Geometry: final body of the model. Coordinates: model frame, mm. Face numbers are marked on the shaded views. Give positions to 0.01 mm unless a question says otherwise; leave off trailing zeros. Write each loop counter-clockwise with the first axis right and the second up, starting at its lowest first coordinate (ties: lowest second). Pieces come first, ordered by that corner, then holes. Notation, with made-up numbers: M -27,76 L 30,76 A27 ccw 30,101 Z; hole C 13.25,-30 d9. An arc over 180 degrees is marked long. Use a Markdown table: item, result. Add a question column.
1) Section A-A on y = 0. Return the cut outline in (x, z).
2) Line query: line 1 (Z direction, x = 3, y = 1.2); line 2 (X direction, y = 1, z = 0.85); line 3 (X direction, y = -0.15, z = 1.1). Output: solid intervals per line, ascending.
3) Draft query along X for the marked faces 1, 2 and 3. Return one class per face: +X half, -X half, draft (parallel to the pull), parting line (faces both ways), or undercut.
4) Section C-C on z = 0.35. Return the cut outline in (x, y).
5) Pin query (flat end, axial travel): pin 1 (0.9 mm diameter, centred on x = 2.5, y = 0, fed in from +Z). Return the tip coordinate at first contact, or that it passes through.
6) Section D-D on x = 0.75. Return the cut outline in (y, z), then the cut area to 3 significant figures.
7) Section B-B on x = 8.75. Return the cut outline in (y, z).
Autodesk Inventor part; units mm, degrees
ref_plane "YZ Plane" through (0, 0, 0) normal (1, 0, 0) x (0, 1, 0)
ref_plane "XZ Plane" through (0, 0, 0) normal (0, 1, 0) x (-1, 0, 0)
ref_plane "XY Plane" through (0, 0, 0) normal (0, 0, 1) x (1, 0, 0)
sketch "草图1" plane through (0, 0, 0) normal (0, 0, 1) x (1, 0, 0)
  line L0 (-8.5, 0) -> (8.5, 0) construction
  line L1 (-8.5, -1.5) -> (8.5, -1.5)
  line L2 (8.5, 1.5) -> (-8.5, 1.5)
  arc A0 (-8.5, 1.5) -> (-8.5, -1.5) centre (-8.5, 0) ccw
  arc A1 (8.5, -1.5) -> (8.5, 1.5) centre (8.5, 0) ccw
  line L3 (5.8209, 0) -> (8.4219, 0) construction
  line L4 (5.8209, -1.1995) -> (8.4219, -1.1995)
  line L5 (8.4219, 1.1995) -> (5.8209, 1.1995)
  arc A2 (5.8209, 1.1995) -> (5.8209, -1.1995) centre (5.8209, 0) ccw
  arc A3 (8.4219, -1.1995) -> (8.4219, 1.1995) centre (8.4219, 0) ccw
  line L6 (0, 2.5577) -> (0, -3.2218)
  line L7 (-5.8209, 0) -> (-8.4219, 0) construction
  line L8 (-5.8209, -1.1995) -> (-8.4219, -1.1995)
  line L9 (-8.4219, 1.1995) -> (-5.8209, 1.1995)
  arc A4 (-5.8209, -1.1995) -> (-5.8209, 1.1995) centre (-5.8209, 0) ccw
  arc A5 (-8.4219, 1.1995) -> (-8.4219, -1.1995) centre (-8.4219, 0) ccw
  point P0 (0, 0)
  point P1 (-10, 0)
  point P2 (10, 0)
  point P3 (7.1214, 0)
  point P4 (4.6214, 0)
  point P5 (9.6214, 0)
  point P6 (-7.1214, 0)
  point P7 (-4.6214, 0)
  point P8 (-9.6214, 0)
  dimension "d0" = 20
  dimension "d1" = 3
  dimension "d2" = 5
extrude "拉伸1" add sketch "草图1" along normal blind 1
extrude "拉伸2" add sketch "草图1" along normal blind 1.5 contours A2 L5 A3 L4 | L8 A5 L9 A4
properties part number "音量接口"
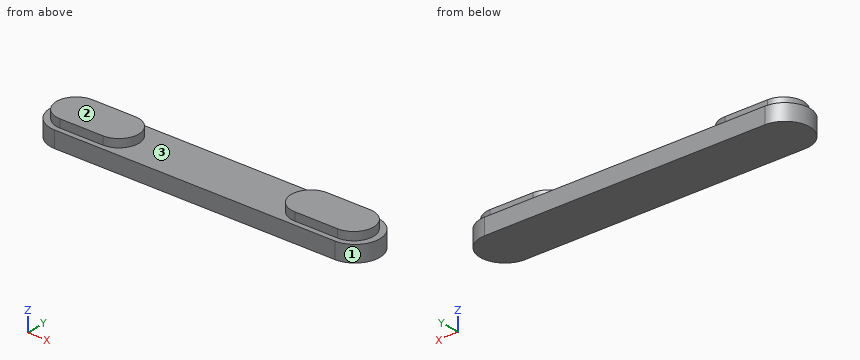
Found:
| question | item | result |
|---|---|---|
| 1 | outline | M -10,0 L 10,0 L 10,1 L 9.62,1 L 9.62,1.5 L 4.62,1.5 L 4.62,1 L -4.62,1 L -4.62,1.5 L -9.62,1.5 L -9.62,1 L -10,1 Z |
| 2 | line 1 | 0 to 1 |
| 2 | line 2 | -9.62 to 9.62 |
| 2 | line 3 | -9.61 to -4.63, 4.63 to 9.61 |
| 3 | face 1 | +X half |
| 3 | face 2 | draft |
| 3 | face 3 | undercut |
| 4 | outline | M -8.5,-1.5 L 8.5,-1.5 A1.5 ccw 8.5,1.5 L -8.5,1.5 A1.5 ccw Z |
| 5 | pin 1 | z = 1 |
| 6 | outline | M -1.5,0 L 1.5,0 L 1.5,1 L -1.5,1 Z |
| 6 | area | 3.00 mm² |
| 7 | outline | M -1.48,0 L 1.48,0 L 1.48,1 L 1.15,1 L 1.15,1.5 L -1.15,1.5 L -1.15,1 L -1.48,1 Z |
